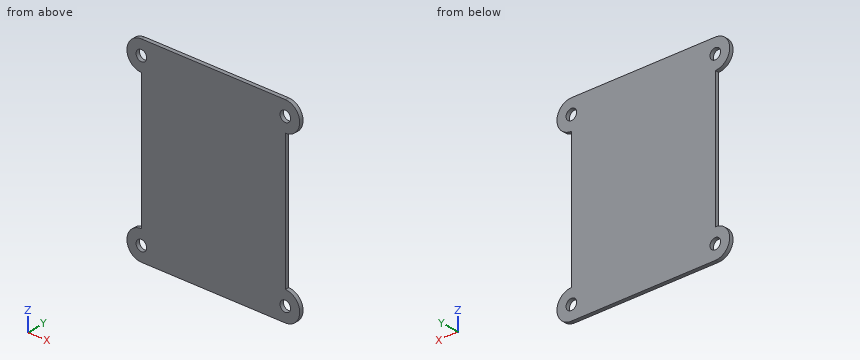
Autodesk Inventor part; units mm, degrees
ref_plane "YZ Plane" through (0, 0, 0) normal (1, 0, 0) x (0, 1, 0)
ref_plane "XZ Plane" through (0, 0, 0) normal (0, 1, 0) x (-1, 0, 0)
ref_plane "XY Plane" through (0, 0, 0) normal (0, 0, 1) x (1, 0, 0)
sketch "スケッチ1" plane through (0, 0, 0) normal (0, 1, 0) x (-1, 0, 0)
  line L0 (15, 20) -> (-15, 20)
  line L1 (-15, 20) -> (-15, -20)
  line L2 (-15, -20) -> (15, -20)
  line L3 (15, -20) -> (15, 14)
  arc A0 (15, 14) -> (15, 20) centre (15, 17) ccw
  line L4 (0, -20) -> (0, 20)
  line L5 (15, 0) -> (-15, 0)
  line L6 (15, 14) -> (15, 20) construction
  circle A1 centre (15, 17) radius 1.1
  arc A2 (15, 20) -> (15, 14) centre (15, 17) ccw construction
  point P0 (0, 0)
  point P1 (0, 0)
  dimension "d0" = 30
  dimension "d1" = 40
  dimension "d2" = 6
  dimension "d3" = 2.2
extrude "押し出し1" add sketch "スケッチ1" along normal blind 0.8 contours A0 L3 L5 L4 L0
mirror "ミラー1" about plane through (0, 0, 20) normal (1, 0, 0) of "押し出し1"
mirror "ミラー2" about plane through (0, 0, 0) normal (0, 0, -1) of "押し出し1", "ミラー1"
properties part number "kiban"
Geometry check sheet. Reference: the model listing, model coordinates, mm. Round coordinates to 2 decimals unless told otherwise and drop trailing zeros. Order: outer loops, then holes, each group sorted by start corner. A loop starts at its lowest first (then second) coordinate and runs counter-clockwise, first axis right, second up. Notation, with made-up numbers: M -2.75,73 L 19.25,73 A8 ccw 19.25,88 Z; hole C 26.5,75.5 d10. An arc over 180 degrees is marked long. Answer in a Markdown table with one row per item.
(1) Sectioned sample at A-A, the plane z = -17. Record the cut outline in (x, y).
Responses:
| item | result |
|---|---|
| outline | M -18,0 L -16.1,0 L -16.1,0.8 L -18,0.8 Z; M -13.9,0 L 13.9,0 L 13.9,0.8 L -13.9,0.8 Z; M 16.1,0 L 18,0 L 18,0.8 L 16.1,0.8 Z |
(2) Sectioned sample at B-B, the plane y = 0.6. Record the cut outline in (x, z), and give its area (3 significant figures).
Responses:
| item | result |
|---|---|
| outline | M -15,-20 L 15,-20 A3 ccw 15,-14 L 15,14 A3 ccw 15,20 L -15,20 A3 ccw -15,14 L -15,-14 A3 ccw Z; hole C -15,-17 d2.2; hole C -15,17 d2.2; hole C 15,-17 d2.2; hole C 15,17 d2.2 |
| area | 1,240 mm² |
(3) Sectioned sample at C-C, the plane z = 2. Record the cut outline in (x, y).
Responses:
| item | result |
|---|---|
| outline | M -15,0 L 15,0 L 15,0.8 L -15,0.8 Z |
(4) Go/stop test with a flat-tipped pin: P1, Ø3, axis at x = 7.5, z = 5.5, coming from the -Y side. Record where the tip stops, or that it passes through.
Responses:
| item | result |
|---|---|
| P1 | stops at y = 0 |
(5) Scan lines: probe 1 along X at (y, z) = (0.2, -17); probe 2 along X at (y, z) = (0.6, 18); probe 3 along X at (y, z) = (0.5, -13.5). Record each from-to range of solid material in increasing order. Write a range as from..to.
Responses:
| item | result |
|---|---|
| probe 1 | x = -18..-16.1, -13.9..13.9, 16.1..18 |
| probe 2 | x = -17.83..-15.46, -14.54..14.54, 15.46..17.83 |
| probe 3 | x = -15..15 |
